Geometry check sheet. Reference: drawing and pictorial views, mm from the part's lowest x, y, z. A direction names the side the tool comes from. Give positions to 0.01 mm unless a question says otherwise; leave off trailing zeros. Write each loop counter-clockwise with the first axis right and the second up, starting at its lowest first coordinate (ties: lowest second). Pieces come first, ordered by that corner, then holes. Notation, with made-up numbers: (69, 77) -> (76, 77) arc R25 ccw to (76, 116) -> close; hole circle Ø10 at (10.25, 63). An arc over 180 degrees is marked (long way). Return JSON: item names as keys, results as strings.
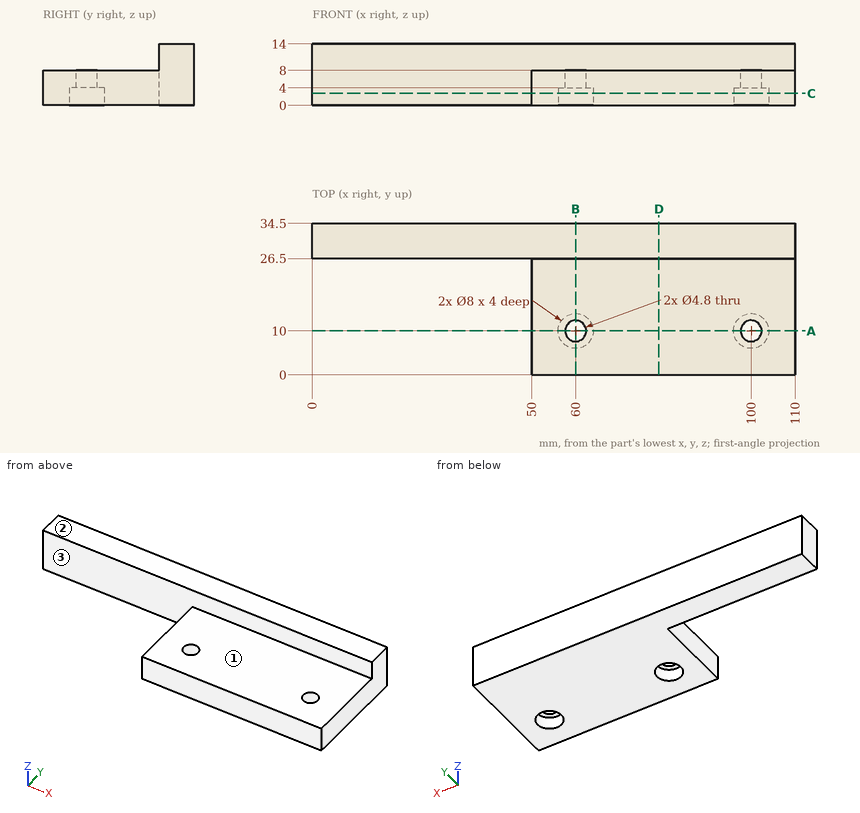
(1) Cross-section at D-D on x = 79. Enter the section's corners in (y, z), then the cut area to 3 significant figures.
Reply:
{"outline": "(0, 0) -> (34.5, 0) -> (34.5, 14) -> (26.5, 14) -> (26.5, 8) -> (0, 8) -> close", "area": "324 mm^2"}
(2) Cross-section at C-C on z = 2.75. Enter the section's corners in (x, y).
Reply:
{"outline": "(0, 26.5) -> (50, 26.5) -> (50, 0) -> (110, 0) -> (110, 34.5) -> (0, 34.5) -> close; hole circle Ø8 at (60, 10); hole circle Ø8 at (100, 10)"}
(3) Set-up check for the marked faces 1, 2 and 3: record each of +Z, -Z, +X, -X, +Y, -Y from which the full face is reachable in a straight line by a thin tool's end or side.
Reply:
{"face 1": "+Z, +X, -X, -Y", "face 2": "+Z, +X, -X, +Y, -Y", "face 3": "+Z, -X, -Y"}
(4) Cross-section at B-B on x = 60. Enter the section's corners in (y, z).
Reply:
{"outline": "(0, 0) -> (6, 0) -> (6, 4) -> (7.6, 4) -> (7.6, 8) -> (0, 8) -> close; (12.4, 4) -> (14, 4) -> (14, 0) -> (34.5, 0) -> (34.5, 14) -> (26.5, 14) -> (26.5, 8) -> (12.4, 8) -> close"}
(5) Thickness scan on L1, parallel to Y at x = 60, z = 1; L2, parallel to X at y = 24, z = 2.5; L3, parallel to Z at x = 51, y = 19. Record the ranges inside material, lowest first.
Reply:
{"L1": "0 to 6, 14 to 34.5", "L2": "50 to 110", "L3": "0 to 8"}
(6) Cross-section at A-A on y = 10. Enter the section's corners in (x, z), then the cut area to 3 significant figures.
Reply:
{"outline": "(50, 0) -> (56, 0) -> (56, 4) -> (57.6, 4) -> (57.6, 8) -> (50, 8) -> close; (62.4, 4) -> (64, 4) -> (64, 0) -> (96, 0) -> (96, 4) -> (97.6, 4) -> (97.6, 8) -> (62.4, 8) -> close; (102.4, 4) -> (104, 4) -> (104, 0) -> (110, 0) -> (110, 8) -> (102.4, 8) -> close", "area": "378 mm^2"}
(7) Depth check by flat-ended pin: pin 1 Ø7 at (x, y) = (60, 10) entering from +Z; pin 2 Ø4 at (x, z) = (68, 10.5) entering from -Y; pin 3 Ø6.5 at (y, z) = (12.5, 5.5) entering from -X. Enter the tip coordinate at first touch or a pass-through.
Reply:
{"pin 1": "z = 8", "pin 2": "y = 26.5", "pin 3": "x = 50"}
